Read the model definition and answer for the solid it produces. Units are mm, in the model's axes. A direction names the side the tool comes from. Give positions to 0.01 mm unless a question says otherwise; leave off trailing zeros. Write each loop counter-clockwise with the first axis right and the second up, starting at its lowest first coordinate (ties: lowest second). Pieces come first, ordered by that corner, then holes. Notation, with made-up numbers: M 14,36 L 38,36 A29 cw 38,56 Z; hole C 10,21.5 d2. An arc over 180 degrees is marked long. Use a Markdown table: item, result. Add a question column.
Item 1: The mould has two halves that part along Y. Classify faces 4 (the cylindrical face through (-1.73, -7.81, 1.48)), 5 (the cylindrical face through (-0.9, -4.05, 1.52)), 6 (the flat face through (5, -2, 0)): pulls with the +Y half, pulls with the -Y half, needs draft (parallel to the pull), parting line crosses it, or undercut.
Item 2: A cutting plane is placed at C-C on y = -4.5. Determine the outline of the cut face in (x, z), then the cut area to 3 significant figures.
Item 3: For faces 1 (the flat face through (5, -2, 3)), 2 (the cylindrical face through (4.91, -1.55, 0.2)), 3 (the cylindrical face through (4.91, 1.55, 2.8)), determine the directions among +Z, -Z, +X, -X, +Y, -Y from which every point of the face is accessible in a straight line to the end or side of a thin tool.
Item 4: Given P1, Ø1.5, axis at x = 4.5, z = 1.5, coming from the +Y side; P2, Ø1.5, axis at x = -1, z = 0.5, coming from the +Y side, each flat-ended and moving along its own axis, determine where each tip first touches the part or whether it passes through.
Item 5: A cutting plane is placed at D-D on y = 6.75. Determine the outline of the cut face in (x, z), then the cut area to 3 significant figures.
Item 6: Consider probe 1 along Y at (x, z) = (0, 1.7); probe 2 along Y at (x, z) = (0, 2.8); probe 3 along X at (y, z) = (-3.75, 1). Determine where each line is inside the solid, lowest interval first. Write a range as [from, to].
Item 7: A cutting plane is placed at A-A on y = 0. Determine the outline of the cut face in (x, z), then the cut area to 3 significant figures.
from build123d import *

# Parameters (mm, degrees)
F0_R     = 8
F1_DEPTH = 3
F2_R     = 4.15
F3_DEPTH = 25
F4_R     = 5.15
F5_DEPTH = 0.4
F6_R     = 5.15
F7_DEPTH = 0.4


with BuildPart() as f1:
    # F0 (on Top) → F1 (new body)
    with BuildSketch(Plane.XY):
        Circle(F0_R)
    extrude(amount=F1_DEPTH)

    # F2 (on face) → F3 (cut)
    with BuildSketch(Plane.XY.offset(3)):
        Circle(F2_R)
    extrude(amount=-F3_DEPTH, mode=Mode.SUBTRACT)

    # F4 (on face) → F5 (cut)
    with BuildSketch(Plane(origin=(0, 0, 0), x_dir=(1, 0, 0), z_dir=(0, 0, -1))):
        Circle(F4_R)
    extrude(amount=-F5_DEPTH, mode=Mode.SUBTRACT)

    # F6 (on face) → F7 (cut)
    with BuildSketch(Plane.XY.offset(3)):
        Circle(F6_R)
    extrude(amount=-F7_DEPTH, mode=Mode.SUBTRACT)


solid = f1.part
Filled in:
| question | item | result |
|---|---|---|
| 1 | face 4 | parting line crosses it |
| 1 | face 5 | undercut |
| 1 | face 6 | needs draft |
| 2 | outline | M -6.61,0 L -2.5,0 L -2.5,0.4 L 2.5,0.4 L 2.5,0 L 6.61,0 L 6.61,3 L 2.5,3 L 2.5,2.6 L -2.5,2.6 L -2.5,3 L -6.61,3 Z |
| 2 | area | 35.7 mm² |
| 3 | face 1 | +Z, +X, -X, +Y, -Y |
| 3 | face 2 | -Z |
| 3 | face 3 | +Z |
| 4 | P1 | y = 7.07 |
| 4 | P2 | y = 8 |
| 5 | outline | M -4.29,0 L 4.29,0 L 4.29,3 L -4.29,3 Z |
| 5 | area | 25.8 mm² |
| 6 | probe 1 | [-8, -4.15], [4.15, 8] |
| 6 | probe 2 | [-8, -5.15], [5.15, 8] |
| 6 | probe 3 | [-7.07, -1.78], [1.78, 7.07] |
| 7 | outline | M -8,0 L -5.15,0 L -5.15,0.4 L -4.15,0.4 L -4.15,2.6 L -5.15,2.6 L -5.15,3 L -8,3 Z; M 4.15,0.4 L 5.15,0.4 L 5.15,0 L 8,0 L 8,3 L 5.15,3 L 5.15,2.6 L 4.15,2.6 Z |
| 7 | area | 21.5 mm² |
